Design review of the part shown in the three views and the two pictorial views. Dimensions are in mm from the part's minimum x, y and z. Coordinates: 2 decimals unless noted, no trailing zeros. Loops run counter-clockwise (first coordinate to the right, second up) from the corner with the lowest first, then second, coordinate; pieces in that order, holes last. Notation, with made-up numbers: (-1, 59.25) -> (31, 59.25) arc R10 cw to (31, 71.25) -> close; hole circle Ø11 at (58, 62.25). An arc over 180 degrees is marked (long way). Use a Markdown table: item, result. Add a question column.
Q1. For probe 1 along Y at (x, z) = (112, 1.2); probe 2 along X at (y, z) = (9.5, 2.6); probe 3 along Y at (x, z) = (87, 2.45), list the stretches that pass through material, from the lowest coordinate up.
Q2. Take a section at C-C on x = 27.5. Write out the cut boundary in (y, z), plus the area to 3 significant figures.
Q3. Take a section at A-A on z = 2.4. Write out the cut boundary in (x, y), plus the area to 3 significant figures.
Q4. Take a section at B-B on x = 87. Write out the cut boundary in (y, z), plus the area to 3 significant figures.
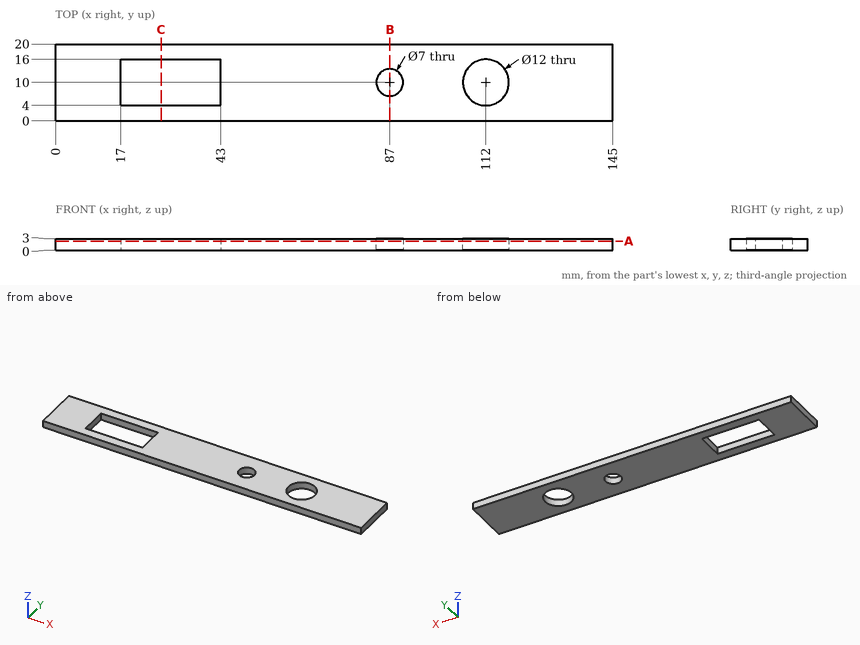
Answer list:
| question | item | result |
|---|---|---|
| 1 | probe 1 | 0 to 4, 16 to 20 |
| 1 | probe 2 | 0 to 17, 43 to 83.54, 90.46 to 106.02, 117.98 to 145 |
| 1 | probe 3 | 0 to 6.5, 13.5 to 20 |
| 2 | outline | (0, 0) -> (4, 0) -> (4, 3) -> (0, 3) -> close; (16, 0) -> (20, 0) -> (20, 3) -> (16, 3) -> close |
| 2 | area | 24.0 mm² |
| 3 | outline | (0, 0) -> (145, 0) -> (145, 20) -> (0, 20) -> close; hole (17, 4) -> (43, 4) -> (43, 16) -> (17, 16) -> close; hole circle Ø7 at (87, 10); hole circle Ø12 at (112, 10) |
| 3 | area | 2,440 mm² |
| 4 | outline | (0, 0) -> (6.5, 0) -> (6.5, 3) -> (0, 3) -> close; (13.5, 0) -> (20, 0) -> (20, 3) -> (13.5, 3) -> close |
| 4 | area | 39.0 mm² |
